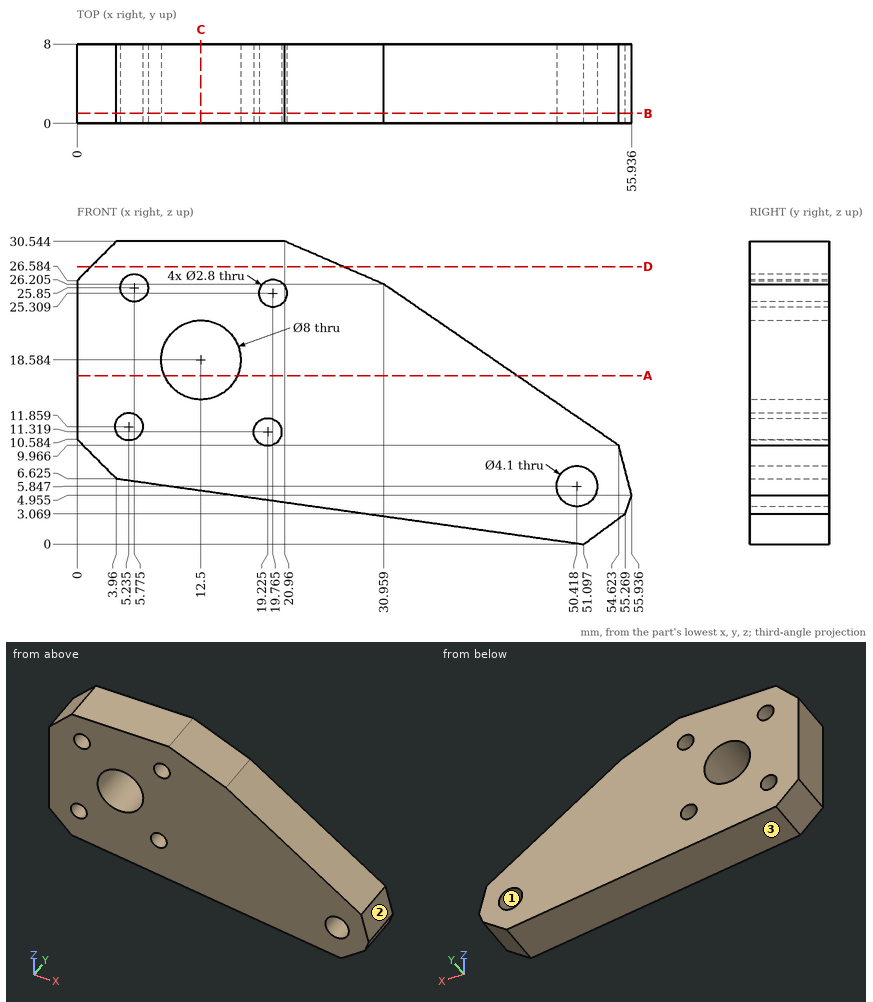
For this review, use the dimensioned drawing (mm, ordinates from the lowest corner) and the shaded views. Give positions to 0.01 mm unless a question says otherwise; leave off trailing zeros. Order: outer loops, then holes, each group sorted by start corner. A loop starts at its lowest first (then second) coordinate and runs counter-clockwise, first axis right, second up.
1) The part is to be moulded in two halves that separate along Z. For the marked faces 1, 2 and 3, say which applies: released by +Z, released by -Z, zero draft, split by the parting line, or undercut.
2) Wall thickness on line 1 (X direction, y = 4.75, z = 25) (1 decimal); line 2 (X direction, y = 5.25, z = 11) (1 decimal); line 3 (X direction, y = 5.25, z = 21) (1 decimal): over which ranges is each line inside the solid? List them lowest first.
3) Take a section at B-B (y = 1). State how many separate pieces and enclosed holes the cut face has, then the cut area to 3 significant figures.
4) Take a section at C-C (x = 12.5). Give the boundary of the cut face in (y, z) (1 decimal), then the cut area to 3 significant figures.
5) Insertion check: pin 1 (2 mm diameter, centred on x = 16.5, y = 6.5, fed in from -Z). The pin has a flat end and moves straight along its axis. Give the tip position at first contact, or say it passes through.
6) Take a section at D-D (z = 28). Give the boundary of the cut face in (x, y) (1 decimal).
7) Take a section at A-A (z = 17). Give the boundary of the cut face in (x, y).
Derived:
1. face 1: undercut
1. face 2: released by +Z
1. face 3: released by -Z
2. line 1: x = 0 to 4.7, 6.9 to 18.4, 21.1 to 32.7
2. line 2: x = 0 to 4.1, 6.3 to 17.9, 20.6 to 53.1
2. line 3: x = 0 to 9.3, 15.7 to 38.5
3. separate pieces: 1
3. enclosed holes: 6
3. area: 1,070 mm2
4. outline: (0, 5.4) - (8, 5.4) - (8, 14.6) - (0, 14.6) - close; (0, 22.6) - (8, 22.6) - (8, 30.5) - (0, 30.5) - close
4. area: 137 mm2
5. pin 1: stops at z = 4.72
6. outline: (1.4, 0) - (26.8, 0) - (26.8, 8) - (1.4, 8) - close
7. outline: (0, 0) - (8.83, 0) - (8.83, 8) - (0, 8) - close; (16.17, 0) - (44.37, 0) - (44.37, 8) - (16.17, 8) - close
